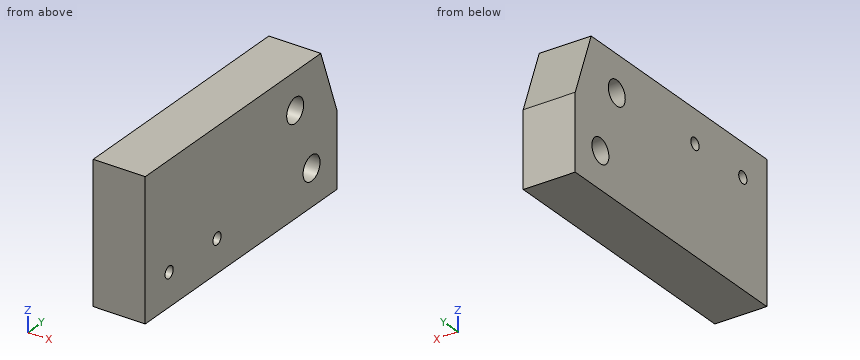
```python
from build123d import *

# Parameters (mm, degrees)
SKETCH1_W                        = 28.575
SKETCH1_H                        = 76.2
BOSS_EXTRUDE1_DEPTH              = 152.4
F_1_2_CLEARANCE_HOLE1_D          = 13.49248
TAP_DRILL_FOR_5_16_18_TAP1_D     = 6.5278
TAP_DRILL_FOR_5_16_18_TAP1_DEPTH = 12.7
TAP_DRILL_FOR_5_16_18_TAP1_TIP   = 1.961148974
TAP_DRILL_FOR_5_16_18_TAP2_D     = 6.5278
TAP_DRILL_FOR_5_16_18_TAP2_DEPTH = 12.7
TAP_DRILL_FOR_5_16_18_TAP2_TIP   = 1.961148974
CUT_EXTRUDE1_DEPTH               = 173.767851827


with BuildPart() as part:
    # Sketch1 → Boss-Extrude1 (new body)
    with BuildSketch(Plane(origin=(0, 0, 0), x_dir=(1, 0, 0), z_dir=(0, 1, 0))):
        with Locations((14.2875, 38.1)):
            Rectangle(SKETCH1_W, SKETCH1_H)
    extrude(amount=BOSS_EXTRUDE1_DEPTH)

    # 1/2 Clearance Hole1 (through all)
    with Locations(Plane(origin=(28.575, 119.317250344, -20.198855574), x_dir=(0, 0, 1), z_dir=(1, 0, 0))):
        with Locations((0, 0), (-35.802288852, -13.030967461)):
            Hole(F_1_2_CLEARANCE_HOLE1_D / 2)

    # Tap Drill for 5/16-18 Tap1
    with Locations(Plane(origin=(28.575, 0, 0), x_dir=(0, 0, -1), z_dir=(1, 0, 0))):
        with Locations((58.1, 57.15), (58.1, 19.05)):
            Hole(TAP_DRILL_FOR_5_16_18_TAP1_D / 2, depth=TAP_DRILL_FOR_5_16_18_TAP1_DEPTH)
            with Locations((0, 0, -(TAP_DRILL_FOR_5_16_18_TAP1_DEPTH + TAP_DRILL_FOR_5_16_18_TAP1_TIP / 2))):  # 118° drill point
                Cone(0, TAP_DRILL_FOR_5_16_18_TAP1_D / 2, TAP_DRILL_FOR_5_16_18_TAP1_TIP, mode=Mode.SUBTRACT)

    # Tap Drill for 5/16-18 Tap2
    with Locations(Plane.ZY):
        with Locations((-18.1, 57.15), (-18.1, 19.05)):
            Hole(TAP_DRILL_FOR_5_16_18_TAP2_D / 2, depth=TAP_DRILL_FOR_5_16_18_TAP2_DEPTH)
            with Locations((0, 0, -(TAP_DRILL_FOR_5_16_18_TAP2_DEPTH + TAP_DRILL_FOR_5_16_18_TAP2_TIP / 2))):  # 118° drill point
                Cone(0, TAP_DRILL_FOR_5_16_18_TAP2_D / 2, TAP_DRILL_FOR_5_16_18_TAP2_TIP, mode=Mode.SUBTRACT)

    # Sketch12 → Cut-Extrude1 (cut, through all)
    with BuildSketch(Plane.ZY):
        Polygon((-34.892963227, 152.4), (0, 139.7), (0, 152.4), align=None)
    extrude(amount=-CUT_EXTRUDE1_DEPTH, mode=Mode.SUBTRACT)


solid = part.part
```
Could you check a few things on this model? Use its own coordinates, in mm. Round coordinates to 2 decimals unless told otherwise and drop trailing zeros. Write each loop counter-clockwise with the first axis right and the second up, starting at its lowest first coordinate (ties: lowest second). Pieces come first, ordered by that corner, then holes.
(1) If I drill on probe 1 along Y at (x, z) = (4.25, -18.1); probe 2 along Z at (x, y) = (8.25, 57.15); probe 3 along Y at (x, z) = (23.75, -59), over which ranges is the centre line in solid material (lowest first)?
Findings below:
probe 1: y = 0 to 15.79, 22.31 to 53.89, 60.41 to 112.91, 125.73 to 146.29
probe 2: z = -76.2 to -21.36, -14.84 to 0
probe 3: y = 0 to 15.91, 22.19 to 54.01, 60.29 to 126.31, 138.39 to 152.4
(2) Suppose I cut it at B-B on z = -10. Write out the boundary of the cut face in (x, y) (3 decimals), and give its area (3 significant figures).
Findings below:
outline: (0, 0) - (28.575, 0) - (28.575, 143.34) - (0, 143.34) - close
area: 4,100 mm2
(3) Suppose I cut it at A-A on x = 8.5. Write out the boundary of the cut face in (y, z), and give its area (3 significant figures).
Findings below:
outline: (0, -76.2) - (152.4, -76.2) - (152.4, -34.89) - (139.7, 0) - (0, 0) - close; hole circle Ø6.53 at (19.05, -18.1); hole circle Ø6.53 at (57.15, -18.1); hole circle Ø13.49 at (119.32, -20.2); hole circle Ø13.49 at (132.35, -56)
area: 11,000 mm2
(4) For pin 1 (4 mm diameter, centred on y = 19.05, z = -18.1, fed in from -X), with a flat end and sliding along its axis, tell me the tip position at first contact or that it passes through.
Findings below:
pin 1: stops at x = 13.46
